Check sheet for the drawn part. Datum: minimum x, y, z corner. Units: mm. Give positions to 0.01 mm unless a question says otherwise; leave off trailing zeros. Loops run counter-clockwise (first coordinate to the right, second up) from the corner with the lowest first, then second, coordinate; pieces in that order, holes last.
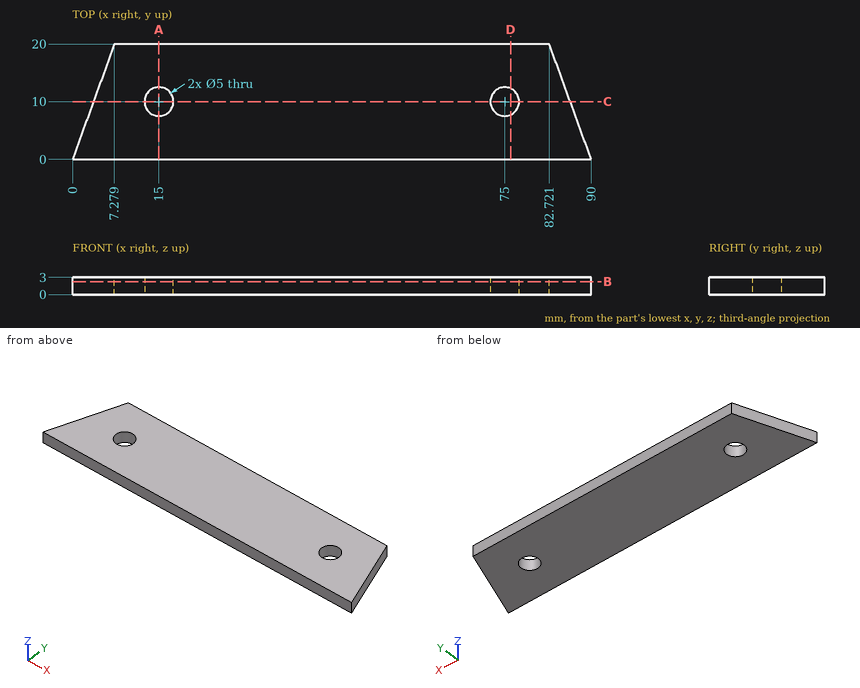
(1) Section check D-D on x = 76. Record the boundary of the cut face in (y, z).
(2) Section check A-A on x = 15. Record the boundary of the cut face in (y, z), plus the area to 3 significant figures.
(3) Section check C-C on y = 10. Record the boundary of the cut face in (x, z).
(4) Material ranges on line 1 (Y direction, x = 15, z = 1.8); line 2 (X direction, y = 9, z = 2.6) (1 decimal); line 3 (X direction, y = 11.25, z = 0.5) (1 decimal), recorded low to high.
(5) Section check B-B on z = 2.25. Record the boundary of the cut face in (x, y), plus the area to 4 significant figures.
(6) Gauge pin test, flat end, axial feed: pin 1 Ø1.5 at (y, z) = (4.5, 1) entering from -X (1 decimal). Record the tip position at first contact, or that the pin passes through.
Computed values:
1. outline: (0, 0) - (7.71, 0) - (7.71, 3) - (0, 3) - close; (12.29, 0) - (20, 0) - (20, 3) - (12.29, 3) - close
2. outline: (0, 0) - (7.5, 0) - (7.5, 3) - (0, 3) - close; (12.5, 0) - (20, 0) - (20, 3) - (12.5, 3) - close
2. area: 45.0 mm2
3. outline: (3.64, 0) - (12.5, 0) - (12.5, 3) - (3.64, 3) - close; (17.5, 0) - (72.5, 0) - (72.5, 3) - (17.5, 3) - close; (77.5, 0) - (86.36, 0) - (86.36, 3) - (77.5, 3) - close
4. line 1: y = 0 to 7.5, 12.5 to 20
4. line 2: x = 3.3 to 12.7, 17.3 to 72.7, 77.3 to 86.7
4. line 3: x = 4.1 to 12.8, 17.2 to 72.8, 77.2 to 85.9
5. outline: (0, 0) - (90, 0) - (82.72, 20) - (7.28, 20) - close; hole circle Ø5 at (15, 10); hole circle Ø5 at (75, 10)
5. area: 1,615 mm2
6. pin 1: stops at x = 1.4
